from build123d import *

# Parameters (mm, degrees)
BOSS_EXTRUDE1_DEPTH = 6


with BuildPart() as part:
    # Sketch1 → Boss-Extrude1 (new body)
    with BuildSketch(Plane.XY):
        with BuildLine():
            Line((-76.2, 131.982271537), (-304.8, 527.929086147))
            ThreePointArc((-304.8, 527.929086147), (-522.857356911, 313.420395513), (-609.271827676, 20))
            Line((-609.271827676, 20), (-151.081964509, 20))
            ThreePointArc((-151.081964509, 20), (-126.685753471, 84.714106662), (-76.2, 131.982271537))
        make_face()
        with BuildLine():
            Line((-335.2, 199.966608393), (-516.736885171, 304.143307511))
            ThreePointArc((-516.736885171, 304.143307511), (-574.388040835, 172.042258023), (-598.849029389, 30))
            Line((-598.849029389, 30), (-335.2, 30))
            Line((-335.2, 30), (-335.2, 199.966608393))
        make_face(mode=Mode.SUBTRACT)
        with BuildLine():
            Line((-330.207563047, 208.631242188), (-511.591783696, 312.720333293))
            ThreePointArc((-511.591783696, 312.720333293), (-422.199493266, 425.755502473), (-308.418556675, 514.196610158))
            Line((-308.418556675, 514.196610158), (-181.552122678, 294.457500701))
            Line((-181.552122678, 294.457500701), (-330.207563047, 208.631242188))
        make_face(mode=Mode.SUBTRACT)
        with BuildLine():
            Line((-89.706166951, 135.375638912), (-176.552122678, 285.797246663))
            Line((-176.552122678, 285.797246663), (-325.2, 199.975354677))
            Line((-325.2, 199.975354677), (-325.2, 30))
            Line((-325.2, 30), (-159.605012453, 30))
            ThreePointArc((-159.605012453, 30), (-135.333005446, 89.770471966), (-89.706166951, 135.375638912))
        make_face(mode=Mode.SUBTRACT)
    extrude(amount=BOSS_EXTRUDE1_DEPTH)


solid = part.part
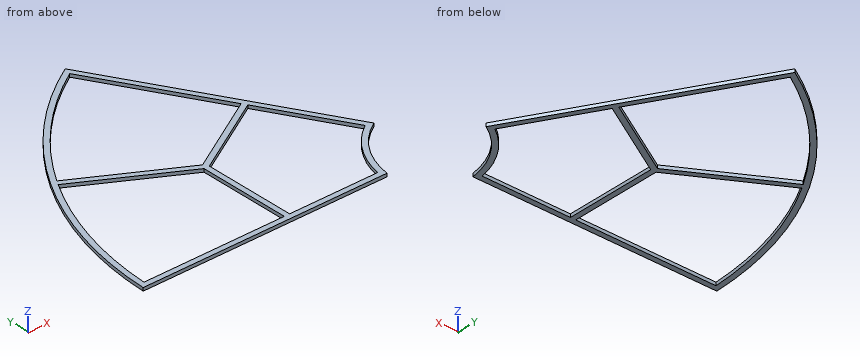
Verification items for the finished model (mm, model axes). Round coordinates to 2 decimals unless told otherwise and drop trailing zeros. Write each loop counter-clockwise with the first axis right and the second up, starting at its lowest first coordinate (ties: lowest second). Pieces come first, ordered by that corner, then holes.
(1) Section check C-C (x = -211.5). Enter the section's corners in (y, z).
Returned:
outline: (20, 0) - (30, 0) - (30, 6) - (20, 6) - close; (265.62, 0) - (277.17, 0) - (277.17, 6) - (265.62, 6) - close; (346.33, 0) - (366.33, 0) - (366.33, 6) - (346.33, 6) - close
(2) Section check B-B (y = 222.5). Enter the section's corners in (x, z).
Returned:
outline: (-567.54, 0) - (-556.79, 0) - (-556.79, 6) - (-567.54, 6) - close; (-374.47, 0) - (-354.38, 0) - (-354.38, 6) - (-374.47, 6) - close; (-306.19, 0) - (-286.19, 0) - (-286.19, 6) - (-306.19, 6) - close; (-140.01, 0) - (-128.46, 0) - (-128.46, 6) - (-140.01, 6) - close
(3) Section check D-D (y = 90). Enter the section's corners in (x, z).
Returned:
outline: (-602.92, 0) - (-592.81, 0) - (-592.81, 6) - (-602.92, 6) - close; (-335.2, 0) - (-325.2, 0) - (-325.2, 6) - (-335.2, 6) - close; (-135.18, 0) - (-122.99, 0) - (-122.99, 6) - (-135.18, 6) - close
(4) Section check A-A (z = 2.5). Enter the section's corners in (x, y), plus the area to 3 significant figures.
Returned:
outline: (-609.27, 20) - (-151.08, 20) arc R152.4 cw to (-76.2, 131.98) - (-304.8, 527.93) arc R609.6 ccw to start; hole (-598.85, 30) - (-335.2, 30) - (-335.2, 199.97) - (-516.74, 304.14) arc R599.6 ccw to start; hole (-511.59, 312.72) - (-330.21, 208.63) - (-181.55, 294.46) - (-308.42, 514.2) arc R599.6 ccw to start; hole (-325.2, 30) - (-159.61, 30) arc R162.4 cw to (-89.71, 135.38) - (-176.55, 285.8) - (-325.2, 199.98) - close
area: 21,900 mm2
(5) Material ranges on line 1 (Y direction, x = -229.5, z = 4); line 2 (Y direction, x = -267, z = 5.7); line 3 (X direction, y = 193, z = 1.05), recorded low to high.
Returned:
line 1: y = 20 to 30, 255.23 to 266.77, 377.51 to 397.51
line 2: y = 20 to 30, 233.58 to 245.12, 442.46 to 462.46
line 3: x = -578.24 to -567.69, -335.2 to -325.2, -122.98 to -111.43
(6) Depth check by flat-ended pin: pin 1 Ø3 at (y, z) = (138, 3) entering from -X; pin 2 Ø3 at (y, z) = (397.5, 3.5) entering from +X. Enter the tip coordinate at first touch or a pass-through.
Returned:
pin 1: stops at x = -594.12
pin 2: stops at x = -228.63
